```python
from build123d import *

# Parameters (mm, degrees)
F1_DEPTH       = 15.5
F2_R           = 25
F3_DEPTH       = 3.5
F5_D           = 3.3
F5_CBORE_D     = 6.5
F5_CBORE_DEPTH = 3
F6_T1_DEPTH    = 12
F6_T3_DEPTH    = 15.5


# Not quite as in the source:
# - a fillet or chamfer that OpenCascade refuses, or shapes differently, is made with other operations: its cross-section is extruded or revolved along the edge and cut away or added


with BuildPart() as f1:
    # F0 (on Top) → F1 (new body)
    with BuildSketch(Plane.XY):
        with BuildLine():
            ThreePointArc((27.1408006584, 24.4054694612), (31.0773430331, 31.0773430331), (24.4054694612, 27.1408006584))
            ThreePointArc((24.4054694612, 27.1408006584), (17.2024322308, 32.1920226973), (9, 35.3730123116))
            Line((9, 35.3730123116), (9, 40))
            Line((9, 40), (-36.5, 40))
            Line((-36.5, 40), (-36.5, 0))
            ThreePointArc((-36.5, 0), (-34.0799737678, -13.0692535358), (-27.1408006584, -24.4054694612))
            ThreePointArc((-27.1408006584, -24.4054694612), (-31.0773430331, -31.0773430331), (-24.4054694612, -27.1408006584))
            ThreePointArc((-24.4054694612, -27.1408006584), (25.8093975133, -25.8093975133), (27.1408006584, 24.4054694612))
        make_face()
    extrude(amount=F1_DEPTH)

    # F2 (on face) → F3 (cut)
    with BuildSketch(Plane(origin=(0, 0, 0), x_dir=(1, 0, 0), z_dir=(0, 0, -1))):
        with BuildLine():
            ThreePointArc((-27.1408006584, 24.4054694612), (-25.8093975133, 25.8093975133), (-24.4054694612, 27.1408006584))
            ThreePointArc((-24.4054694612, 27.1408006584), (-31.0773430331, 31.0773430331), (-27.1408006584, 24.4054694612))
        make_face()
        with BuildLine():
            ThreePointArc((27.1408006584, -24.4054694612), (25.8093975133, -25.8093975133), (24.4054694612, -27.1408006584))
            ThreePointArc((24.4054694612, -27.1408006584), (31.0773430331, -31.0773430331), (27.1408006584, -24.4054694612))
        make_face()
        Circle(F2_R)
    extrude(amount=-F3_DEPTH, mode=Mode.SUBTRACT)

    # F5 (through all)
    with Locations(Plane.XY.offset(15.5)):
        with Locations((-28.2489159084, -28.2489159084), (28.2489159084, 28.2489159084)):
            CounterBoreHole(F5_D / 2, F5_CBORE_D / 2, F5_CBORE_DEPTH)

    # F6: fillet of radius 5 on 5 edges, made by hand

    # F6_s2 → F6_t1 (join)
    with BuildSketch(Plane.XY.offset(3.5)):
        with BuildLine():
            ThreePointArc((-30.783749931, -19.6114951033), (-30.0157488678, -22.6856125629), (-31.2497097164, -25.6040649633))
            ThreePointArc((-31.2497097164, -25.6040649633), (-29.369056893, -24.4089570317), (-27.1408006584, -24.4054694612))
            ThreePointArc((-27.1408006584, -24.4054694612), (-29.0612962165, -22.0837284492), (-30.783749931, -19.6114951033))
        make_face()
        with BuildLine():
            ThreePointArc((-19.6114951033, -30.783749931), (-22.6856125629, -30.0157488678), (-25.6040649633, -31.2497097164))
            ThreePointArc((-25.6040649633, -31.2497097164), (-24.4089570317, -29.369056893), (-24.4054694612, -27.1408006584))
            ThreePointArc((-24.4054694612, -27.1408006584), (-22.0837284492, -29.0612962165), (-19.6114951033, -30.783749931))
        make_face()
        with BuildLine():
            ThreePointArc((30.783749931, 19.6114951033), (30.0157488678, 22.6856125629), (31.2497097164, 25.6040649633))
            ThreePointArc((31.2497097164, 25.6040649633), (29.369056893, 24.4089570317), (27.1408006584, 24.4054694612))
            ThreePointArc((27.1408006584, 24.4054694612), (29.0612962165, 22.0837284492), (30.783749931, 19.6114951033))
        make_face()
        with BuildLine():
            ThreePointArc((19.6114951033, 30.783749931), (22.6856125629, 30.0157488678), (25.6040649633, 31.2497097164))
            ThreePointArc((25.6040649633, 31.2497097164), (24.4089570317, 29.369056893), (24.4054694612, 27.1408006584))
            ThreePointArc((24.4054694612, 27.1408006584), (22.0837284492, 29.0612962165), (19.6114951033, 30.783749931))
        make_face()
    extrude(amount=F6_T1_DEPTH)

    # F6_s4 → F6_t3 (join)
    with BuildSketch(Plane.XY):
        with BuildLine():
            ThreePointArc((12.313253012, 34.3603521557), (9.9113734005, 36.189206534), (9, 39.0672497112))
            Line((9, 39.0672497112), (9, 35.3730123116))
            ThreePointArc((9, 35.3730123116), (10.6686483978, 34.9060158334), (12.313253012, 34.3603521557))
        make_face()
    extrude(amount=F6_T3_DEPTH)


solid = f1.part
```
CAD build for the part. Positions are in the model's coordinates, mm. A direction names the side the tool comes from. Round coordinates to 2 decimals unless told otherwise and drop trailing zeros. Write each loop counter-clockwise with the first axis right and the second up, starting at its lowest first coordinate (ties: lowest second). Pieces come first, ordered by that corner, then holes. Notation, with made-up numbers: (7, -37) - (42, -37) arc R35 cw to (42, 0) - close; hole circle Ø6 at (-16.5, 40.5). An arc over 180 degrees is marked (long way). Write item = value, one per line. Start each with the question number.
Q1. Which spindle directions (+Z, -Z, +X, -X, +Y, -Y) get a long thin tool onto all of the face, cutting with end or side? Do faces 1 (the flat face through (26, 27, 3.5)), 2 (the flat face through (-26, -28, 3.5)), 3 (the cylindrical face through (23.846, -7.509, 1.726)), 4 (the flat face through (-30, -27, 12.5)). Say none if no direction does.
Q2. Band-saw the part on D-D (x = 28). Give the cut face in (y, z).
Q3. Band-saw the part on C-C (y = -13). Give the cut face in (x, z).
Q4. Mould opens along Y. For faces 5 (the flat face through (-13, 40, 8)), 6 (the flat face through (-36.5, 20, 8)), 7 (the cylindrical face through (25, 28.39, 14.02)) say: pulls with the +Y half, pulls with the -Y half, needs draft (parallel to the pull), parting line crosses it, or undercut.
Q5. Band-saw the part on A-A (x = 0). Give the cut face in (y, z), then the cut area to 3 significant figures.
Q6. Probe L1, parallel to X at y = 0, z = 1.8; L2, parallel to Y at x = 0, z = 1.75; L3, parallel to X at y = 28.5, z = 4. List the from-to ranges inside material, lowest first. Write a range as from..to.
Q7. Band-saw the part on B-B (z = 8). Give the cut face in (x, y), then the cut area to 3 significant figures.
Q8. Drop flat-ended pins along their axis: pin 1 (5 mm diameter, centred on y = 7.5, z = 9.5, fed in from +X); pin 2 (6 mm diameter, centred on x = 28.25, y = 28.25, fed in from -Z); pin 3 (2 mm diameter, centred on x = 28, y = 29, fed in from +Z); pin 4 (2.5 mm diameter, centred on x = 28.25, y = 28.25, fed in from -Z). Give the stop position or say it passes through.
Answers below:
q1.face_1 = -Z, +X, +Y
q1.face_2 = -Z, -X, -Y
q1.face_3 = -Z
q1.face_4 = +Z
q2.outline = (-23.41, 0) - (23.41, 0) - (23.41, 3.5) - (26.62, 3.5) - (26.62, 12.5) - (25.01, 12.5) - (25.01, 15.5) - (-23.41, 15.5) - close; (29.88, 3.5) - (32.24, 3.5) - (32.24, 15.5) - (31.49, 15.5) - (31.49, 12.5) - (29.88, 12.5) - close
q3.outline = (-34.11, 0) - (-21.35, 0) - (-21.35, 3.5) - (21.35, 3.5) - (21.35, 0) - (34.11, 0) - (34.11, 15.5) - (-34.11, 15.5) - close
q4.face_5 = pulls with the +Y half
q4.face_6 = needs draft
q4.face_7 = undercut
q5.outline = (-36.5, 0) - (-25, 0) - (-25, 3.5) - (25, 3.5) - (25, 0) - (40, 0) - (40, 15.5) - (-36.5, 15.5) - close
q5.area = 1,010 mm2
q6.L1 = -36.5..-25, 25..36.5
q6.L2 = -36.5..-25, 25..40
q6.L3 = -36.5..26.62, 29.88..32.24
q7.outline = (-36.5, 0) arc R36.5 ccw to (-30.78, -19.61) arc R5 cw to (-31.25, -25.6) arc R4 ccw to (-25.6, -31.25) arc R5 cw to (-19.61, -30.78) arc R36.5 ccw to (30.78, 19.61) arc R5 cw to (31.25, 25.6) arc R4 ccw to (25.6, 31.25) arc R5 cw to (19.61, 30.78) arc R36.5 ccw to (12.31, 34.36) arc R5 cw to (9, 39.07) - (9, 40) - (-36.5, 40) - close; hole circle Ø3.3 at (-28.25, -28.25); hole circle Ø3.3 at (28.25, 28.25)
q7.area = 4,740 mm2
q8.pin_1 = 36.16
q8.pin_2 = 3.5
q8.pin_3 = 12.5
q8.pin_4 = through
